Could you check a few things on this drawing? It's one solid part, dimensions in mm from its lowest x, y, z. Give positions to 0.01 mm unless a question says otherwise; leave off trailing zeros. Write each loop counter-clockwise with the first axis right and the second up, starting at its lowest first coordinate (ties: lowest second). Pieces come first, ordered by that corner, then holes. Notation, with made-up numbers: M 72,6.5 L 77,6.5 A22 cw 77,34.5 Z; hole C -33.5,9.5 d9. An arc over 180 degrees is marked long. Answer as CSV lines item,"result". Start each with the question number.
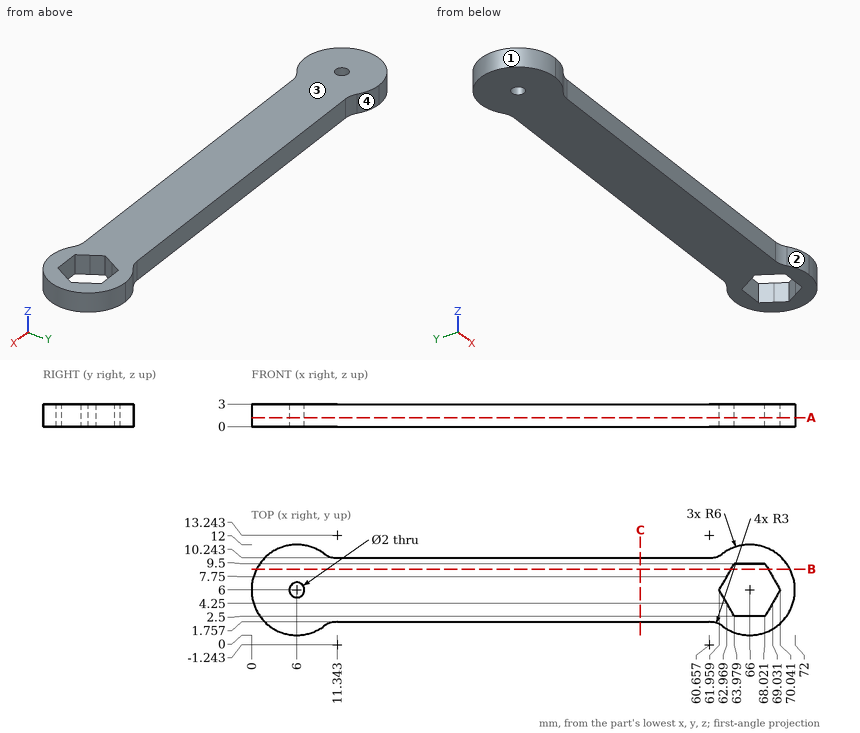
1) I want a section at B-B, the plane y = 8.75. Please give me the cut outline in (x, z), then the cut area to 3 significant figures.
2) I want a section at C-C, the plane x = 51.5. Please give me the cut outline in (y, z).
3) Thinking about a two-plate mould opening in X: for the marked faces 1, 2, 3 and 4, which applies, released by +X, released by -X, zero draft, split by the parting line, or undercut?
4) I need wall thicknesses on L1, parallel to Y at x = 6, z = 1.3; L2, parallel to Y at x = 41, z = 0.45; L3, parallel to X at y = 7.25, z = 1.9. Which ranges of each line are inside material? Lowest first, please. Write a range as from..to.
5) I want a section at A-A, the plane z = 1.2. Please give me the cut outline in (x, y).
6) I'm going to push flat-ended pins straight in: P1, Ø1.2, axis at x = 6, y = 6, coming from the -Z side; P2, Ø1.5, axis at x = 40, z = 2, coming from the -Y side. Where does each tip first touch, or does it pass through?
Values found:
1,outline,"M 0.67,0 L 63.55,0 L 63.55,3 L 0.67,3 Z; M 68.45,0 L 71.33,0 L 71.33,3 L 68.45,3 Z"
1,area,"197 mm²"
2,outline,"M 1.76,0 L 10.24,0 L 10.24,3 L 1.76,3 Z"
3,face 1,"released by -X"
3,face 2,"undercut"
3,face 3,"zero draft"
3,face 4,"undercut"
4,L1,"y = 0..5, 7..12"
4,L2,"y = 1.76..10.24"
4,L3,"x = 0.13..62.68, 69.32..71.87"
5,outline,"M 6,0 A6 ccw 9.56,1.17 A3 cw 11.34,1.76 L 60.66,1.76 A3 cw 62.44,1.17 A6 ccw 66,0 A6 ccw 66,12 A6 ccw 62.44,10.83 A3 cw 60.66,10.24 L 11.34,10.24 A3 cw 9.56,10.83 A6 ccw 6,12 A6 ccw Z; hole C 6,6 d2; hole M 61.96,6 L 63.98,2.5 L 68.02,2.5 L 70.04,6 L 68.02,9.5 L 63.98,9.5 Z"
6,P1,"passes through"
6,P2,"stops at y = 1.76"
